from build123d import *

# Parameters (mm, degrees)
SKETCH012_R             = 12.85
PAD006_DEPTH            = 4
SKETCH013_R             = 11
POCKET004_DEPTH         = 0.5
SKETCH014_R             = 6
PAD007_DEPTH            = 3.5
SKETCH016_R             = 1.5
PAD008_DEPTH            = 6.5
SKETCH015_R             = 4
POCKET005_DEPTH         = 7.001
SKETCH017_R             = 2.6
PAD009_DEPTH            = 4
BODY002_PLACEMENT_ANGLE = 90


with BuildPart() as part:
    # Sketch012 → Pad006 (new body)
    with BuildSketch(Plane.XY):
        Circle(SKETCH012_R)
    extrude(amount=PAD006_DEPTH)

    # Sketch013 → Pocket004 (cut)
    with BuildSketch(Plane.XY.offset(4)):
        Circle(SKETCH013_R)
    extrude(amount=-POCKET004_DEPTH, mode=Mode.SUBTRACT)

    # Sketch014 (on Face5 of Pocket004) → Pad007 (join)
    with BuildSketch(Plane.XY.offset(3.5)):
        Circle(SKETCH014_R)
    extrude(amount=PAD007_DEPTH)

    # Sketch016 → Pad008 (join)
    with BuildSketch(Plane.XZ):
        with Locations((0, 5)):
            Circle(SKETCH016_R)
    extrude(amount=PAD008_DEPTH)

    # Sketch015 (on Face7 of Pad007) → Pocket005 (cut, through all)
    with BuildSketch(Plane.XY.offset(7)):
        Circle(SKETCH015_R)
    extrude(amount=-POCKET005_DEPTH, mode=Mode.SUBTRACT)

    # Sketch017 → Pad009 (join)
    with BuildSketch(Plane.XY):
        with BuildLine():
            Line((-3.542445, 13.25), (4.373404, 13.25))
            ThreePointArc((7.251161, 12.477086), (5.863276, 13.053407), (4.373404, 13.25))
            Line((7.251161, 12.477086), (21.969939, 3.956011))
            ThreePointArc((23.65, 1.04209), (23.1999, 2.72387), (21.969939, 3.956011))
            Line((23.65, 1.04209), (23.65, -1.322208))
            ThreePointArc((21.959502, -4.246432), (23.196964, -3.011059), (23.65, -1.322208))
            Line((8.3652, -12.074699), (21.959502, -4.246432))
            ThreePointArc((3.969015, -13.25), (6.244305, -12.951104), (8.3652, -12.074699))
            Line((3.969015, -13.25), (-2.715889, -13.25))
            ThreePointArc((-8.759411, -11.630643), (-5.844246, -12.838144), (-2.715889, -13.25))
            Line((-21.777636, -4.114568), (-8.759411, -11.630643))
            ThreePointArc((-23.65, -0.871538), (-23.148302, -2.743902), (-21.777636, -4.114568))
            Line((-23.65, -0.871538), (-23.65, 1.686966))
            ThreePointArc((-22.483817, 3.706854), (-23.337522, 2.853149), (-23.65, 1.686966))
            Line((-8.043592, 12.043921), (-22.483817, 3.706854))
            ThreePointArc((-3.542445, 13.25), (-5.87241, 12.943254), (-8.043592, 12.043921))
        make_face()
        with Locations((-18.5, -0.045589)):
            Circle(SKETCH017_R, mode=Mode.SUBTRACT)
        with Locations((19.5, 0)):
            Circle(SKETCH017_R, mode=Mode.SUBTRACT)
    extrude(amount=-PAD009_DEPTH)


with BuildPart() as part_1:
    # Body002 placement: moved
    add(part.part.moved(Location((-58, 0, 4))).rotate(Axis((-58, 0, 4), (0, 0, 1)), BODY002_PLACEMENT_ANGLE))


solid = part_1.part
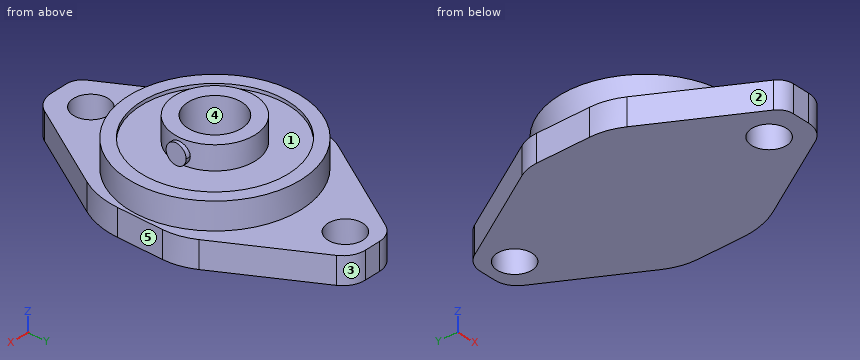
Design review of the part built by this model. Coordinates are the model's own, in mm. Face numbers are marked on the shaded views. A direction names the side the tool comes from. Coordinates: 2 decimals unless noted, no trailing zeros. Write each loop counter-clockwise with the first axis right and the second up, starting at its lowest first coordinate (ties: lowest second). Pieces come first, ordered by that corner, then holes. Notation, with made-up numbers: (-36, 37) -> (6, 37) arc R21 cw to (6, 49) -> close; hole circle Ø11 at (27.25, 34.25). An arc over 180 degrees is marked (long way). Write each question's results on one line, items separated by ' | '. Start each with the question number.
(1) For line 1 along Y through (x, z) = (-58, 7.75); line 2 along X through (y, z) = (-18.5, 2.6); line 3 along X through (y, z) = (0, 7.25), list the stretches that pass through material, from the lowest coordinate up. Write a range as from..to.
(2) Take a section at B-B on z = 2.5. Write out the cut boundary in (x, y).
(3) Take a section at A-A on y = 19.5. Write out the cut boundary in (x, z).
(4) Take a section at D-D on x = -50.5. Write out the cut boundary in (y, z), and give its area (3 significant figures).
(5) Take a section at C-C on x = -58.5. Write out the cut boundary in (y, z).
(6) The part is to be moulded in two halves that separate along X. For the marked faces 1, 2 and 3, say which applies: pulls with the +X half, pulls with the -X half, needs draft (parallel to the pull), parting line crosses it, or undercut.
(7) Tool access review of the marked faces 4 and 5: name each direction out of +Z, -Z, +X, -X, +Y, -Y from which nothing blocks a thin tool from reaching the whole face with its end or side.
(8) Clearance check with flat-ended pins moving along their axes: P1, Ø1.5, axis at x = -52.5, y = 18, coming from the +Z side; P2, Ø6, axis at y = 11.5, z = 4.5, coming from the -X side; P3, Ø2.5, axis at y = -0.5, z = 9, coming from the +X side. State where each tip first meets the part, or that it passes through.
Results found:
1) line 1: y = -12.85..-11, -6..-4, 4..6, 11..12.85 | line 2: x = -64.01..-60.55, -55.35..-51.99 | line 3: x = -70.85..-62, -54..-45.15
2) outline: (-71.25, -3.54) arc R9 ccw to (-70.04, -8.04) -> (-61.71, -22.48) arc R2.33 ccw to (-59.69, -23.65) -> (-57.13, -23.65) arc R3.74 ccw to (-53.89, -21.78) -> (-46.37, -8.76) arc R12.09 ccw to (-44.75, -2.72) -> (-44.75, 3.97) arc R8.81 ccw to (-45.93, 8.37) -> (-53.75, 21.96) arc R3.37 ccw to (-56.68, 23.65) -> (-59.04, 23.65) arc R3.37 ccw to (-61.96, 21.97) -> (-70.48, 7.25) arc R5.74 ccw to (-71.25, 4.37) -> close; hole circle Ø5.2 at (-58, 19.5); hole circle Ø5.2 at (-57.95, -18.5)
3) outline: (-63.39, 0) -> (-60.6, 0) -> (-60.6, 4) -> (-63.39, 4) -> close; (-55.4, 0) -> (-52.34, 0) -> (-52.34, 4) -> (-55.4, 4) -> close
4) outline: (-15.91, 0) -> (16.31, 0) -> (16.31, 4) -> (10.43, 4) -> (10.43, 8) -> (8.05, 8) -> (8.05, 7.5) -> (-8.05, 7.5) -> (-8.05, 8) -> (-10.43, 8) -> (-10.43, 4) -> (-15.91, 4) -> close | area: 204 mm2
5) outline: (-23.65, 0) -> (-21.04, 0) -> (-21.04, 4) -> (-23.65, 4) -> close; (-15.96, 0) -> (16.95, 0) -> (16.95, 4) -> (12.84, 4) -> (12.84, 8) -> (10.99, 8) -> (10.99, 7.5) -> (5.98, 7.5) -> (5.98, 11) -> (3.97, 11) -> (3.97, 4) -> (-3.97, 4) -> (-3.97, 11) -> (-5.98, 11) -> (-5.98, 7.5) -> (-10.99, 7.5) -> (-10.99, 8) -> (-12.84, 8) -> (-12.84, 4) -> (-15.96, 4) -> close; (22.05, 0) -> (23.65, 0) -> (23.65, 4) -> (22.05, 4) -> close
6) face 1: undercut | face 2: pulls with the -X half | face 3: pulls with the +X half
7) face 4: +Z | face 5: +Z, -Z, +X, +Y, -Y
8) P1: stops at z = 4 | P2: stops at x = -69.73 | P3: stops at x = -45.15
